```python
from build123d import *

# Parameters (mm, degrees)
CUT_EXTRUDE1_DEPTH = 1.3
CHAMFER1_SIZE      = 0.3


with BuildPart() as part:
    # Sketch1 → Revolve1 (revolve)
    with BuildSketch(Plane.XY, mode=Mode.PRIVATE) as revolve1_sk:
        Polygon((0, 1.5), (12, 1.5), (12, 0), (-3, 0), (-3, 2.75), (0, 2.75), align=None)
    revolve(revolve1_sk.sketch.rotate(Axis((-3, 0, 0), (1, 0, 0)), 180), axis=Axis((-3, 0, 0), (1, 0, 0)))

    # Sketch2 → Cut-Revolve1 (revolve, cut)
    with BuildSketch(Plane.XY, mode=Mode.PRIVATE) as cut_revolve1_sk:
        Polygon((-0.948924226, 0), (-1.7, 1.25), (-3, 1.25), (-3, 0), align=None)
    revolve(cut_revolve1_sk.sketch.rotate(Axis((-3, 0, 0), (1, 0, 0)), 180), axis=Axis((-3, 0, 0), (1, 0, 0)), mode=Mode.SUBTRACT)

    # Sketch3 → Cut-Extrude1 (cut)
    with BuildSketch(Plane.ZY.offset(3)):
        Polygon((1.25, 0.721687836), (0, 1.443375673), (-1.25, 0.721687836), (-1.25, -0.721687836), (0, -1.443375673), (1.25, -0.721687836), align=None)
    extrude(amount=-CUT_EXTRUDE1_DEPTH, mode=Mode.SUBTRACT)

    # Chamfer1
    chamfer1_edges = [part.edges().sort_by_distance(p)[0] for p in [
        (-3, 2.75, 0),
    ]]
    chamfer(chamfer1_edges, length=CHAMFER1_SIZE)


solid = part.part
```
Source: CAD feature listing. Evaluate the final solid. Frame: model axes, mm. A direction names the side the tool comes from. Round coordinates to 2 decimals unless told otherwise and drop trailing zeros. Loops run counter-clockwise (first coordinate to the right, second up) from the corner with the lowest first, then second, coordinate; pieces in that order, holes last.
1. Mould query, pull axis Y, two halves, no side actions, for faces 4 (the flat face through (-3, 1.1, 1.1)), 5 (the flat face through (-2, 0, 1.25)), 6 (the cylindrical face through (-1.331, 0.596, 2.685)). Classes: released by +Y, released by -Y, zero draft, split by the parting line, or undercut.
2. Ray query, L1, parallel to X at y = 1.7, z = 1.7; L2, parallel to Z at x = 3.5, y = 0.1; L3, parallel to Y at x = 6.75, z = 0.4. Return the intervals inside material, ascending.
3. Section query A-A on x = -1.5. Output: boundary loops of the cut face in (y, z), and give its area (3 significant figures).
4. Contact query for flat-ended pins moving along their axis: pin 1 (2 mm diameter, centred on x = 2.5, y = 0.5, fed in from -Z); pin 2 (1 mm diameter, centred on x = 3, z = 1, fed in from -Y); pin 3 (1 mm diameter, centred on x = 9, z = -1.5, fed in from -Y). Output: stop coordinate, or through.
5. Access query for faces 1 (the flat face through (0, -1.2, 1.2)), 2 (the flat face through (-2.36, 1.08, 0.63)), 3 (the flat face through (12, 0, 0)). Directions: +Z, -Z, +X, -X, +Y, -Y. A direction counts if a zero-diameter tool reaches every point of the face in a straight line with its end or side. Return the directions, or none.
6. Section query B-B on x = 9.25. Output: boundary loops of the cut face in (y, z), and give its area (3 significant figures).
Answers below:
1. face 4: zero draft
1. face 5: undercut
1. face 6: split by the parting line
2. L1: x = -3 to 0
2. L2: z = -1.5 to 1.5
2. L3: y = -1.45 to 1.45
3. outline: circle Ø5.5 at (0, 0); hole circle Ø1.83 at (0, 0)
3. area: 21.1 mm2
4. pin 1: stops at z = -1.5
4. pin 2: stops at y = -1.41
4. pin 3: stops at y = -1.12
5. face 1: +X
5. face 2: -X
5. face 3: +Z, -Z, +X, +Y, -Y
6. outline: circle Ø3 at (0, 0)
6. area: 7.07 mm2
